CAD build for the part. Positions are in the model's coordinates, mm. Face numbers are marked on the shaded views. A direction names the side the tool comes from. Coordinates: 2 decimals unless noted, no trailing zeros. Loops run counter-clockwise (first coordinate to the right, second up) from the corner with the lowest first, then second, coordinate; pieces in that order, holes last. Notation, with made-up numbers: (49, 2.5) -> (61, 2.5) arc R13 ccw to (61, 21.5) -> close; hole circle Ø2 at (26, 56.5). An arc over 180 degrees is marked (long way). Return JSON: item names as keys, results as strings. Group by question number.
(1) Probe L1, parallel to X at y = 0, z = -1.75; L2, parallel to X at y = 14.5, z = -2.75; L3, parallel to Y at x = -3.5, z = -5. List the from-to ranges inside material, lowest first.
(2) Mould opens along X. For the marked faces 3, 4 and 5 say: pulls with the +X half, pulls with the -X half, needs draft (parallel to the pull), parting line crosses it, or undercut.
(3) Saw through at B-B on z = -4.25. Write the cut outline in (x, y), then the cut area to 3 significant figures.
(4) Saw through at A-A on y = 0. Write the cut outline in (x, z).
(5) Tool access for the marked faces 1 and 2: list every direction of +Z, -Z, +X, -X, +Y, -Y with a clear straight run to the whole face (end or side of a thin tool).
(6) Flat gauge pins, fed straight in: pin 1 Ø16 at (x, y) = (3.5, 21) entering from +Z; pin 2 Ø17.5 at (x, y) = (-3.5, 10.5) entering from +Z; pin 3 Ø3 at (y, z) = (3.5, -5) entering from +X; pin 4 Ø1.5 at (y, z) = (7.5, -6.5) entering from +X. Where does each tip first touch, or does it go through?
```python
from build123d import *

# Parameters (mm, degrees)
SKETCH_2_R               = 1.051872146
EXTRUDE_1_DEPTH          = 8
PATTERN_CIRCULAR_1_COUNT = 6
CHAMFER_1_SIZE           = 2


with BuildPart() as part:
    # Эскиз1 → Повернуть1 (revolve)
    with BuildSketch(Plane(origin=(0, 0, 0), x_dir=(1, 0, 0), z_dir=(0, 1, 0))):
        Polygon((-39.012426389, 8.189631494), (-39.012426389, 9.189631494), (-6.012426389, 9.189631494), (-6.012426389, 8.189631494), (-35.012426389, 8.189631494), (-35.012426389, 0.189631494), (-36.012426389, 0.189631494), (-36.012426389, 8.189631494), align=None)
    revolve(axis=Axis((-6.012426389, 0, -9.189631494), (0, 0, 1)))

    # Эскиз2 → Бобышка-Вытянуть1 (add)
    with BuildSketch(Plane.XY.offset(-0.189631494)):
        with Locations((-6.68742643, 29.992405288)):
            Circle(SKETCH_2_R)
    extrude_1 = extrude(amount=-EXTRUDE_1_DEPTH)

    # Круговой массив1: Бобышка-Вытянуть1 ×6 about axis
    pattern_circular_1_axis = Axis((-6.012426389, 0, 0), (0, 0, 1))
    for i in range(1, PATTERN_CIRCULAR_1_COUNT):
        add(extrude_1.rotate(pattern_circular_1_axis, i * 360 / PATTERN_CIRCULAR_1_COUNT))

    # Фаска1
    # the kernel refuses this chamfer: 2 mm, written as the material it takes off along each edge
    with BuildSketch(Plane(origin=(-6.012426389, 0, -8.189631494), x_dir=(-1, 0, 0), z_dir=(0, 1, 0))) as chamfer_1_piece_1_section:
        Polygon((33, -CHAMFER_1_SIZE), (33 - CHAMFER_1_SIZE, 0), (33, 0), align=None)
    chamfer_1_piece_1 = revolve(axis=Axis((-6.012426389, 0, -8.189631494), (0, 0, 1)), mode=Mode.PRIVATE)
    chamfer_1_piece_1 = chamfer_1_piece_1 - Plane(origin=(19.62425849, 15.580769827, -9.135558261), x_dir=(0.5000000000000001, -0.8660254037844386, 0), z_dir=(0, 0, 1)) * Cylinder(1.051872146, 132, mode=Mode.PRIVATE)
    chamfer_1_piece_1 = chamfer_1_piece_1 - Plane(origin=(20.299258531, -14.411635461, -9.135558261), x_dir=(-0.5000000000000004, -0.8660254037844384, 0), z_dir=(0, 0, 1)) * Cylinder(1.051872146, 132, mode=Mode.PRIVATE)
    chamfer_1_piece_1 = chamfer_1_piece_1 - Plane(origin=(-5.337426348, -29.992405288, -9.135558261), x_dir=(-1, 0, 0), z_dir=(0, 0, 1)) * Cylinder(1.051872146, 132, mode=Mode.PRIVATE)
    chamfer_1_piece_1 = chamfer_1_piece_1 - Plane(origin=(-31.649111268, -15.580769827, -9.135558261), x_dir=(-0.49999999999999983, 0.8660254037844388, 0), z_dir=(0, 0, 1)) * Cylinder(1.051872146, 132, mode=Mode.PRIVATE)
    chamfer_1_piece_1 = chamfer_1_piece_1 - Plane(origin=(-32.324111309, 14.411635461, -9.135558261), x_dir=(0.5000000000000001, 0.8660254037844386, 0), z_dir=(0, 0, 1)) * Cylinder(1.051872146, 132, mode=Mode.PRIVATE)
    chamfer_1_piece_1 = chamfer_1_piece_1 - Plane(origin=(-6.68742643, 29.992405288, -9.135558261), x_dir=(1, 0, 0), z_dir=(0, 0, 1)) * Cylinder(1.051872146, 132, mode=Mode.PRIVATE)
    add(chamfer_1_piece_1, mode=Mode.SUBTRACT)


solid = part.part
```
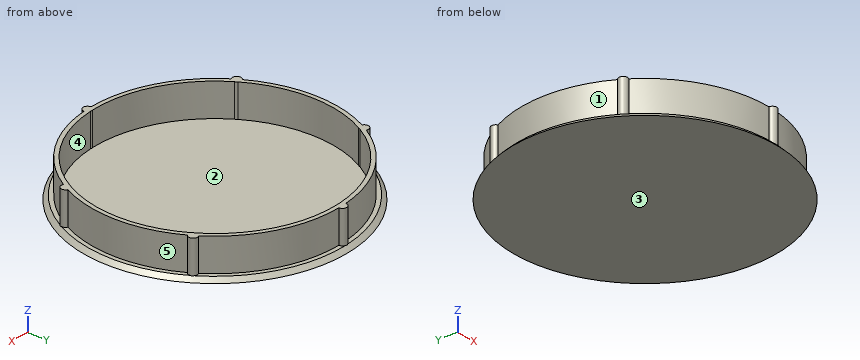
Geometry results:
{
 "1": {"L1": "-36.01 to -35.01, 22.99 to 23.99", "L2": "-33.37 to -31.13, 19.1 to 20.25", "L3": "-29.89 to -28.89, 28.89 to 29.89"},
 "2": {"face 3": "needs draft", "face 4": "undercut", "face 5": "pulls with the +X half"},
 "3": {"outline": "(-32.81, 13.48) arc R30 ccw to (-32.18, -14.67) arc R1.05 ccw (long way) to (-31.09, -16.47) arc R30 ccw to (-6.39, -30) arc R1.05 ccw (long way) to (-4.29, -29.95) arc R30 ccw to (19.78, -15.33) arc R1.05 ccw (long way) to (20.79, -13.48) arc R30 ccw to (20.15, 14.67) arc R1.05 ccw (long way) to (19.06, 16.47) arc R30 ccw to (-5.64, 30) arc R1.05 ccw (long way) to (-7.74, 29.95) arc R30 ccw to (-31.8, 15.33) arc R1.05 ccw (long way) to start; hole (-31.6, 13.65) arc R29 ccw to (-30.96, -14.79) arc R1.05 cw to (-30.63, -15.33) arc R29 ccw to (-5.68, -29) arc R1.05 cw to (-5.04, -28.98) arc R29 ccw to (19.27, -14.21) arc R1.05 cw to (19.57, -13.65) arc R29 ccw to (18.93, 14.79) arc R1.05 cw to (18.6, 15.33) arc R29 ccw to (-6.34, 29) arc R1.05 cw to (-6.99, 28.98) arc R29 ccw to (-31.29, 14.21) arc R1.05 cw to start", "area": "196 mm²"},
 "4": {"outline": "(-38.01, -9.19) -> (25.99, -9.19) -> (24.99, -8.19) -> (23.99, -8.19) -> (23.99, -0.19) -> (22.99, -0.19) -> (22.99, -8.19) -> (-35.01, -8.19) -> (-35.01, -0.19) -> (-36.01, -0.19) -> (-36.01, -8.19) -> (-37.01, -8.19) -> close"},
 "5": {"face 1": "+Z, -X", "face 2": "+Z"},
 "6": {"pin 1": "z = -0.19", "pin 2": "z = -8.19", "pin 3": "x = 23.92", "pin 4": "x = 23.22"}
}
